The listing builds one solid part. Answer for the finished solid, in the listing's coordinates (mm). Round coordinates to 2 decimals unless told otherwise and drop trailing zeros. Order: outer loops, then holes, each group sorted by start corner. A loop starts at its lowest first (then second) coordinate and runs counter-clockwise, first axis right, second up. Notation, with made-up numbers: (16, -24.75) -> (21, -24.75) arc R18 ccw to (21, -12.75) -> close; hole circle Ø11 at (62.25, 33.5). An arc over 180 degrees is marked (long way). Answer in a Markdown table with one row per item. Add a question column.
Autodesk Inventor part; units mm, degrees
ref_plane "YZ Plane" through (0, 0, 0) normal (1, 0, 0) x (0, 1, 0)
ref_plane "XZ Plane" through (0, 0, 0) normal (0, 1, 0) x (-1, 0, 0)
ref_plane "XY Plane" through (0, 0, 0) normal (0, 0, 1) x (1, 0, 0)
sketch "Sketch1" plane through (0, 0, 0) normal (0, 0, 1) x (1, 0, 0)
  line L0 (0, 0) -> (25.4, 0)
  line L1 (25.4, 0) -> (25.4, -50.8)
  line L2 (25.4, -50.8) -> (0, -50.8)
  line L3 (0, -50.8) -> (0, 0)
  line L4 (22.225, -3.175) -> (3.175, -3.175)
  line L5 (3.175, -3.175) -> (3.175, -47.625)
  line L6 (3.175, -47.625) -> (22.225, -47.625)
  line L7 (22.225, -47.625) -> (22.225, -3.175)
  dimension "d0" = 25.4
  dimension "d1" = 50.8
  dimension "d2" = 3.175
extrude "Extrusion1" add sketch "Sketch1" along normal blind 635
sketch "Sketch2" plane through (25.4, -50.8, 0) normal (1, 0, 0) x (0, 0, -1)
  circle A0 centre (-38.1, 25.4) radius 14.2875
  line L0 (0, 50.8) -> (0, 0)
  line L1 (0, 50.8) -> (-635, 50.8)
  circle A1 centre (-148.1252, 25.4) radius 14.2875
  dimension "d5" = 38.1
  dimension "d6" = 25.4
  dimension "d7" = 28.575
  dimension "d8" = 110.0252
  dimension "d9" = 28.575
  dimension "d10" = 25.4
extrude "Extrusion2" cut sketch "Sketch2" against normal blind 25.4
properties part number "DRL Tall"
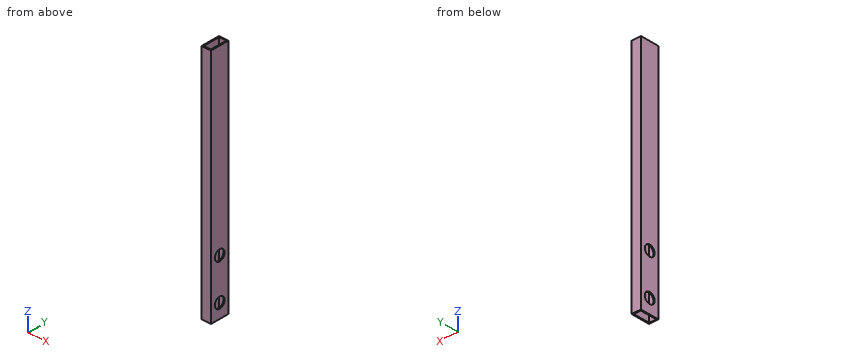
1. The part is cut by section B-B (z = 38.1). Give the vertices of the cut face in (x, y) (1 decimal), then the cut area to 3 significant figures.
2. The part is cut by section A-A (x = 11.25). Give the vertices of the cut face in (y, z) (3 decimals), then the cut area to 3 significant figures.
3. Straight lines are drawn through the part: line 1 along Y through (x, z) = (15.25, 588) (3 decimals); line 2 along X through (y, z) = (-25, 315) (3 decimals); line 3 along Y through (x, z) = (2.1, 38.1). For each, find the intervals that lie inside material, in ascending order.
4. The part is cut by section C-C (y = -25.4). Give the vertices of the cut face in (x, z) (1 decimal).
Report:
| question | item | result |
|---|---|---|
| 1 | outline | (0, -50.8) -> (25.4, -50.8) -> (25.4, -39.7) -> (22.2, -39.7) -> (22.2, -47.6) -> (3.2, -47.6) -> (3.2, -39.7) -> (0, -39.7) -> close; (0, -11.1) -> (3.2, -11.1) -> (3.2, -3.2) -> (22.2, -3.2) -> (22.2, -11.1) -> (25.4, -11.1) -> (25.4, 0) -> (0, 0) -> close |
| 1 | area | 262 mm^2 |
| 2 | outline | (-50.8, 0) -> (-47.625, 0) -> (-47.625, 635) -> (-50.8, 635) -> close; (-3.175, 0) -> (0, 0) -> (0, 635) -> (-3.175, 635) -> close |
| 2 | area | 4,030 mm^2 |
| 3 | line 1 | y = -50.8 to -47.625, -3.175 to 0 |
| 3 | line 2 | x = 0 to 3.175, 22.225 to 25.4 |
| 3 | line 3 | y = -50.8 to -39.69, -11.11 to 0 |
| 4 | outline | (0, 0) -> (3.2, 0) -> (3.2, 23.8) -> (0, 23.8) -> close; (0, 52.4) -> (3.2, 52.4) -> (3.2, 133.8) -> (0, 133.8) -> close; (0, 162.4) -> (3.2, 162.4) -> (3.2, 635) -> (0, 635) -> close; (22.2, 0) -> (25.4, 0) -> (25.4, 23.8) -> (22.2, 23.8) -> close; (22.2, 52.4) -> (25.4, 52.4) -> (25.4, 133.8) -> (22.2, 133.8) -> close; (22.2, 162.4) -> (25.4, 162.4) -> (25.4, 635) -> (22.2, 635) -> close |
